from build123d import *

# Parameters (mm, degrees)
SKETCH1_W           = 78
SKETCH1_H           = 115
BOSS_EXTRUDE1_DEPTH = 4
SKETCH5_R           = 1.4
CUT_EXTRUDE3_DEPTH  = 2
SKETCH6_W           = 3
SKETCH6_H           = 10
BOSS_EXTRUDE3_DEPTH = 41
SKETCH7_R           = 1.5
CUT_EXTRUDE4_DEPTH  = 104.015775491
FILLET1_R           = 2


with BuildPart() as part:
    # Sketch1 → Boss-Extrude1 (new body)
    with BuildSketch(Plane(origin=(0, 0, 0), x_dir=(1, 0, 0), z_dir=(0, 1, 0))):
        Rectangle(SKETCH1_W, SKETCH1_H)
    extrude(amount=BOSS_EXTRUDE1_DEPTH)

    # Sketch5 → Cut-Extrude3 (cut)
    with BuildSketch(Plane(origin=(0, 4, 0), x_dir=(1, 0, 0), z_dir=(0, 1, 0))):
        with Locations(Location((-35.5, 54, 0), (0, 0, 270))):
            Circle(SKETCH5_R)
        with Locations(Location((35.5, 54, 0), (0, 0, 270))):
            Circle(SKETCH5_R)
        with Locations(Location((35.5, -54, 0), (0, 0, 90))):
            Circle(SKETCH5_R)
        with Locations(Location((-35.5, -54, 0), (0, 0, 90))):
            Circle(SKETCH5_R)
    extrude(amount=-CUT_EXTRUDE3_DEPTH, mode=Mode.SUBTRACT)

    # Sketch6 → Boss-Extrude3 (add)
    with BuildSketch(Plane.XZ):
        with Locations((-34.5, 21.55)):
            Rectangle(SKETCH6_W, SKETCH6_H)
        with Locations((34.5, 21.55)):
            Rectangle(SKETCH6_W, SKETCH6_H)
    extrude(amount=BOSS_EXTRUDE3_DEPTH)

    # Sketch7 → Cut-Extrude4 (cut, through all)
    with BuildSketch(Plane(origin=(36, 0, 0), x_dir=(0, 0, -1), z_dir=(1, 0, 0))):
        with Locations((-21.8, -12)):
            Circle(SKETCH7_R)
        with Locations((-21.8, -28)):
            Circle(SKETCH7_R)
    extrude(amount=-CUT_EXTRUDE4_DEPTH, mode=Mode.SUBTRACT)

    # Fillet1
    fillet1_edges = [part.edges().sort_by_distance(p)[0] for p in [
        (-39, 2, -57.5),
        (39, 2, -57.5),
        (39, 2, 57.5),
        (-39, 2, 57.5),
    ]]
    fillet(fillet1_edges, radius=FILLET1_R)


solid = part.part
The listing builds one solid part. Answer for the finished solid, in the listing's coordinates (mm). A direction names the side the tool comes from. Round coordinates to 2 decimals unless told otherwise and drop trailing zeros. Loops run counter-clockwise (first coordinate to the right, second up) from the corner with the lowest first, then second, coordinate; pieces in that order, holes last. Notation, with made-up numbers: M 49,71.5 L 96,71.5 A20 ccw 96,90.5 Z; hole C 65.25,80.25 d4. An arc over 180 degrees is marked long. Return JSON: item names as keys, results as strings.
Q1. Each of these flat-tipped pins is pushed along its axis until it touches: pin 1 Ø8 at (y, z) = (-16.5, 21.5) entering from -X; pin 2 Ø1.8 at (y, z) = (-28, 21.8) entering from +X; pin 3 Ø10 at (x, z) = (20.5, 9.5) entering from -Y; pin 4 Ø1.5 at (x, y) = (34, -21) entering from +Z. Where does it stop, or does it pass through?
Results list:
{"pin 1": "stops at x = -36", "pin 2": "passes through", "pin 3": "stops at y = 0", "pin 4": "stops at z = 26.55"}
Q2. Find section B-B, the plane z = 21.8. Determine the outline of the cut face in (x, y), plus the area to 3 significant figures.
Results list:
{"outline": "M -39,0 L -36,0 L -36,-10.5 L -33,-10.5 L -33,0 L 33,0 L 33,-10.5 L 36,-10.5 L 36,0 L 39,0 L 39,4 L -39,4 Z; M -36,-41 L -33,-41 L -33,-29.5 L -36,-29.5 Z; M -36,-26.5 L -33,-26.5 L -33,-13.5 L -36,-13.5 Z; M 33,-41 L 36,-41 L 36,-29.5 L 33,-29.5 Z; M 33,-26.5 L 36,-26.5 L 36,-13.5 L 33,-13.5 Z", "area": "522 mm2"}
Q3. Find section D-D, the plane z = -54. Determine the outline of the cut face in (x, y).
Results list:
{"outline": "M -39,0 L 39,0 L 39,4 L 36.9,4 L 36.9,2 L 34.1,2 L 34.1,4 L -34.1,4 L -34.1,2 L -36.9,2 L -36.9,4 L -39,4 Z"}
Q4. The mould has two halves that part along Z. Classify faces 1 (the face through (34.32, 3.01, 53.25)), 2 (the face through (-1, 2, 57.5)), 3 (the face through (-1, 4, -1)): released by +Z, released by -Z, zero draft, split by the parting line, or undercut.
Results list:
{"face 1": "undercut", "face 2": "released by +Z", "face 3": "zero draft"}
Q5. Find section C-C, the plane y = -28. Determine the outline of the cut face in (x, z).
Results list:
{"outline": "M -36,16.55 L -33,16.55 L -33,20.3 L -36,20.3 Z; M -36,23.3 L -33,23.3 L -33,26.55 L -36,26.55 Z; M 33,16.55 L 36,16.55 L 36,20.3 L 33,20.3 Z; M 33,23.3 L 36,23.3 L 36,26.55 L 33,26.55 Z"}
Q6. Find the intervals of material crossed by line 1 along Y through (x, z) = (-34, 21.8); line 2 along X through (y, z) = (3, -54); line 3 along Z through (x, y) = (35, 3), in increasing order. Write a range as from..to.
Results list:
{"line 1": "y = -41..-29.5, -26.5..-13.5, -10.5..4", "line 2": "x = -39..-36.9, -34.1..34.1, 36.9..39", "line 3": "z = -57.5..-55.31, -52.69..52.69, 55.31..57.5"}
Q7. Which of the six approach directions +Z, -Z, +X, -X, +Y, -Y give full straight-line access (tool end or side, diameter ignored) to faces 4 (the face through (-36, -20, 21)), 5 (the face through (35, 2, 54)), 6 (the face through (34, -20, 26.55)), 7 (the face through (33, -20, 21))?
Results list:
{"face 4": "+Z, -Z, -X, -Y", "face 5": "+Y", "face 6": "+Z, +X, -X, -Y", "face 7": "+Z, -Z, -Y"}
Q8. Find section A-A, the plane y = -19.5. Determine the outline of the cut face in (x, z), plus the area to 3 significant figures.
Results list:
{"outline": "M -36,16.55 L -33,16.55 L -33,26.55 L -36,26.55 Z; M 33,16.55 L 36,16.55 L 36,26.55 L 33,26.55 Z", "area": "60.0 mm2"}
